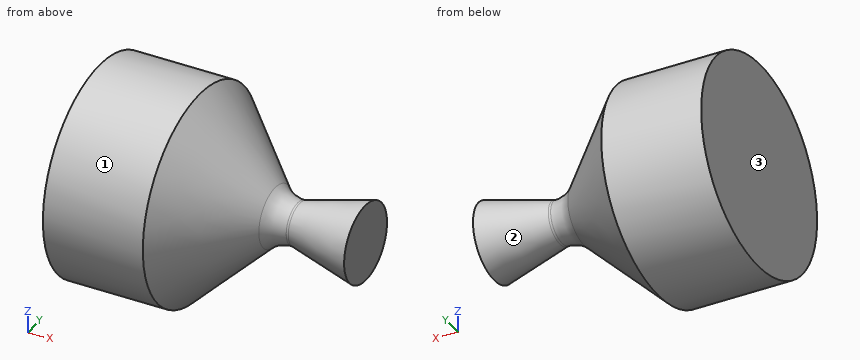
```python
from build123d import *


with BuildPart() as part:
    # Sketch1 → Revolve1 (revolve)
    with BuildSketch(Plane.XY, mode=Mode.PRIVATE) as revolve1_sk:
        with BuildLine():
            Line((-13.36065, 28.0607), (13.36065, 28.0607))
            Line((13.36065, 28.0607), (33.34363095, 8.07771905))
            ThreePointArc((33.34363095, 8.07771905), (36.074675364, 6.252893513), (39.2961619, 5.6121))
            Line((39.2961619, 5.6121), (39.3061619, 5.6121))
            ThreePointArc((39.3061619, 5.6121), (39.599172317, 5.631304917), (39.887169245, 5.688591068))
            Line((39.887169245, 5.688591068), (57.419630863, 10.3864))
            Line((57.419630863, 10.3864), (57.419630863, 0))
            Line((57.419630863, 0), (-13.36065, 0))
            Line((-13.36065, 0), (-13.36065, 28.0607))
        make_face()
    revolve(revolve1_sk.sketch.rotate(Axis((0, 0, 0), (1, 0, 0)), 90), axis=Axis((0, 0, 0), (1, 0, 0)))


solid = part.part
```
Verification items for the finished model (mm, model axes). Face numbers are marked on the shaded views. Give positions to 0.01 mm unless a question says otherwise; leave off trailing zeros. Order: outer loops, then holes, each group sorted by start corner. A loop starts at its lowest first (then second) coordinate and runs counter-clockwise, first axis right, second up. Notation, with made-up numbers: (-9.75, -14) - (22.25, -14) arc R22 cw to (22.25, 13) - close; hole circle Ø8 at (-8.75, 81.25). An arc over 180 degrees is marked (long way). Answer as CSV lines item,"result". Start each with the question number.
Item 1: Gauge pin test, flat ends, axial feed: pin 1 (10 mm diameter, centred on x = 43.5, z = -17, fed in from -Y); pin 2 (5 mm diameter, centred on x = 20.5, z = 14, fed in from +Y); pin 3 (10 mm diameter, centred on y = -14.5, z = -10.5, fed in from +X); pin 4 (12 mm diameter, centred on y = -9, z = 21, fed in from +X). Record the tip position at first contact, or that the pin passes through.
Item 2: Section check D-D, the plane x = 52.5. Record the boundary of the cut face in (y, z).
Item 3: Material ranges on L1, parallel to Z at x = 49, y = 1; L2, parallel to Y at x = -5.5, z = 0.5; L3, parallel to Y at x = -8, z = 1, recorded low to high.
Item 4: Section check C-C, the plane x = 19. Record the boundary of the cut face in (y, z).
Item 5: Mould release check, pull along X, two halves, no side actions. Record for the marked faces 1, 2 and 3: released by +X, released by -X, zero draft, split by the parting line, or undercut.
Filled in:
1,pin 1,"through"
1,pin 2,"y = 19.25"
1,pin 3,"x = 28.52"
1,pin 4,"x = 24.57"
2,outline,"circle Ø18.14 at (0, 0)"
3,L1,"-8.07 to 8.07"
3,L2,"-28.06 to 28.06"
3,L3,"-28.04 to 28.04"
4,outline,"circle Ø44.84 at (0, 0)"
5,face 1,"zero draft"
5,face 2,"undercut"
5,face 3,"released by -X"
